```python
from build123d import *

# Parameters (mm, degrees)
SKETCH1_R           = 3.175
BOSS_EXTRUDE1_DEPTH = 5
SKETCH2_W           = 59.69
SKETCH2_H           = 15
BOSS_EXTRUDE2_DEPTH = 3.81
SKETCH5_R           = 3.175
BOSS_EXTRUDE3_DEPTH = 5


with BuildPart() as part:
    # Sketch1 → Boss-Extrude1 (new body)
    with BuildSketch(Plane.XY):
        with BuildLine():
            Line((-47.217391304, 7.923913043), (28.982608696, 7.923913043))
            ThreePointArc((28.982608696, 7.923913043), (36.482608696, 0.423913043), (28.982608696, -7.076086957))
            Line((28.982608696, -7.076086957), (-47.217391304, -7.076086957))
            ThreePointArc((-47.217391304, -7.076086957), (-54.717391304, 0.423913043), (-47.217391304, 7.923913043))
        make_face()
        with Locations((-47.217391304, 0.423913043)):
            Circle(SKETCH1_R, mode=Mode.SUBTRACT)
        with Locations((28.982608696, 0.423913043)):
            Circle(SKETCH1_R, mode=Mode.SUBTRACT)
    extrude(amount=BOSS_EXTRUDE1_DEPTH)

    # Sketch2 → Boss-Extrude2 (add)
    with BuildSketch(Plane.XY.offset(5)):
        with Locations((-9.117391304, 0.423913043)):
            Rectangle(SKETCH2_W, SKETCH2_H)
    extrude(amount=BOSS_EXTRUDE2_DEPTH)

    # Sketch5 → Boss-Extrude3 (add)
    with BuildSketch(Plane.XY.offset(8.81)):
        with BuildLine():
            Line((-47.217391304, 7.923913043), (28.982608696, 7.923913043))
            ThreePointArc((28.982608696, 7.923913043), (36.482608696, 0.423913043), (28.982608696, -7.076086957))
            Line((28.982608696, -7.076086957), (-47.217391304, -7.076086957))
            ThreePointArc((-47.217391304, -7.076086957), (-54.717391304, 0.423913043), (-47.217391304, 7.923913043))
        make_face()
        with Locations((-47.217391304, 0.423913043)):
            Circle(SKETCH5_R, mode=Mode.SUBTRACT)
        with Locations((28.982608696, 0.423913043)):
            Circle(SKETCH5_R, mode=Mode.SUBTRACT)
    extrude(amount=BOSS_EXTRUDE3_DEPTH)


solid = part.part
```
Can you work these out from the model? Positions are in its coordinate system, mm. A direction names the side the tool comes from. Round coordinates to 2 decimals unless told otherwise and drop trailing zeros. Loops run counter-clockwise (first coordinate to the right, second up) from the corner with the lowest first, then second, coordinate; pieces in that order, holes last. Notation, with made-up numbers: (36, 79) -> (71, 79) arc R25 ccw to (71, 105) -> close; hole circle Ø6 at (41.5, -28.5). An arc over 180 degrees is marked (long way). One line per item, written item: value. Start each with the question number.
1. For pin 1 (1 mm diameter, centred on x = 12, y = -3, fed in from -Z); pin 2 (4 mm diameter, centred on y = -3, z = 6, fed in from +X); pin 3 (8 mm diameter, centred on y = 6, z = 4, fed in from -X); pin 4 (4 mm diameter, centred on y = -1.5, z = 7, fed in from -X), each with a flat end and sliding along its axis, tell me the tip position at first contact or that it passes through.
2. If we section it at B-B, the plane y = -2: Write out the boundary of the cut face in (x, z).
3. For faces 1 (the flat face through (20.728, 0, 7)), 2 (the cylindrical face through (-54.716, 0.259, 11.275)), 3 (the flat face through (-43, 1, 5)), which set-ups out of +Z, -Z, +X, -X, +Y, -Y let a thin tool reach every point of the face, with its end or its side?
4. If we section it at A-A, the plane x = 22: Write out the boundary of the cut face in (y, z), then the cut area to 3 significant figures.
5. If we mould it in two halves opening along X, with no side actions, what happens to faces 4 (the flat face through (-43, 1, 8.81)), 5 (the cylindrical face through (36.48, 0.59, 11.28)), 6 (the cylindrical face through (-50.39, 0.56, 2.46)), 7 (the cylindrical face through (31.916, -0.792, 2.465))? For each: pulls with the +X half, pulls with the -X half, needs draft (parallel to the pull), parting line crosses it, or undercut.
6. If I drill on probe 1 along X at (y, z) = (0.75, 1.5); probe 2 along X at (y, z) = (-0.5, 3) (3 decimals); probe 3 along Z at (x, y) = (31.5, 7.25), over which ranges is the centre line in solid material (lowest first)?
7. If we section it at C-C, the plane z = 2.5: Write out the boundary of the cut face in (x, y) (3 decimals).
8. If we section it at D-D, the plane z = 8: Write out the boundary of the cut face in (x, y), then the cut area to 3 significant figures.
Calculated:
1. pin 1: stops at z = 0
1. pin 2: stops at x = 36.29
1. pin 3: stops at x = -54.55
1. pin 4: stops at x = -54.64
2. outline: (-54.31, 0) -> (-49.27, 0) -> (-49.27, 5) -> (-54.31, 5) -> close; (-54.31, 8.81) -> (-49.27, 8.81) -> (-49.27, 13.81) -> (-54.31, 13.81) -> close; (-45.17, 0) -> (26.93, 0) -> (26.93, 5) -> (20.73, 5) -> (20.73, 8.81) -> (26.93, 8.81) -> (26.93, 13.81) -> (-45.17, 13.81) -> (-45.17, 8.81) -> (-38.96, 8.81) -> (-38.96, 5) -> (-45.17, 5) -> close; (31.03, 0) -> (36.08, 0) -> (36.08, 5) -> (31.03, 5) -> close; (31.03, 8.81) -> (36.08, 8.81) -> (36.08, 13.81) -> (31.03, 13.81) -> close
3. face 1: +X, +Y, -Y
3. face 2: +Z, -Z, -X
3. face 3: -X, +Y, -Y
4. outline: (-7.08, 0) -> (7.92, 0) -> (7.92, 5) -> (-7.08, 5) -> close; (-7.08, 8.81) -> (7.92, 8.81) -> (7.92, 13.81) -> (-7.08, 13.81) -> close
4. area: 150 mm²
5. face 4: needs draft
5. face 5: pulls with the +X half
5. face 6: undercut
5. face 7: undercut
6. probe 1: x = -54.71 to -50.38, -44.06 to 25.82, 32.14 to 36.48
6. probe 2: x = -54.66 to -50.255, -44.18 to 25.945, 32.02 to 36.425
6. probe 3: z = 0 to 5, 8.81 to 13.81
7. outline: (-47.217, -7.076) -> (28.983, -7.076) arc R7.5 ccw to (28.983, 7.924) -> (-47.217, 7.924) arc R7.5 ccw to start; hole circle Ø6.35 at (-47.217, 0.424); hole circle Ø6.35 at (28.983, 0.424)
8. outline: (-38.96, -7.08) -> (20.73, -7.08) -> (20.73, 7.92) -> (-38.96, 7.92) -> close
8. area: 895 mm²
